```python
from build123d import *

# Parameters (mm, degrees)
SALIENTE_EXTRUIR1_DEPTH = 10
SALIENTE_EXTRUIR2_DEPTH = 5
REDONDEO1_R             = 5
CORTAR_EXTRUIR2_REACH   = 48.394
CROQUIS4_R              = 1.5
CORTAR_EXTRUIR3_DEPTH   = 5


with BuildPart() as part:
    # Croquis1 → Saliente-Extruir1 (new, symmetric)
    with BuildSketch(Plane(origin=(0, 0, 0), x_dir=(0, 0, -1), z_dir=(1, 0, 0))):
        Polygon((20.5, 0), (0, 0), (-3.1, -9.2), (-3.1, -13.1), (-3.019721522, -15), (0.873328538, -14.835511509), (0.8, -13.1), (6, -13.1), (6, -10.1), (2.7, -10.1), (2.7, -7), (6, -7), (6, -4), (14, -4), (14, -7), (17.3, -7), (17.3, -10.1), (14, -10.1), (14, -13.1), (20.5, -13.1), align=None)
    extrude(amount=SALIENTE_EXTRUIR1_DEPTH, both=True)

    # Croquis1<4> → Saliente-Extruir2 (add, symmetric)
    with BuildSketch(Plane(origin=(0, 0, 0), x_dir=(0, 0, -1), z_dir=(1, 0, 0))):
        Polygon((0.873328538, -14.835511509), (-3.019721522, -15), (-1.94652503, -40.4), (1.94652503, -40.235511509), align=None)
    extrude(amount=SALIENTE_EXTRUIR2_DEPTH, both=True)

    # Redondeo1
    redondeo1_edges = [part.edges().sort_by_distance(p)[0] for p in [
        (-5, -40.317755755, 0),
        (5, -40.317755755, 0),
    ]]
    fillet(redondeo1_edges, radius=REDONDEO1_R - 0.0001)  # a hair under: the kernel refuses the full size

    # Croquis3 → Cortar-Extruir2 (cut, up to next)
    with BuildSketch(Plane(origin=(0, 0, 0), x_dir=(1, 0, 0), z_dir=(0, 1, 0)), mode=Mode.PRIVATE) as cortar_extruir2_sk1:
        with BuildLine():
            Line((-6, 11.75), (6, 11.75))
            ThreePointArc((6, 11.75), (7.5, 10.25), (6, 8.75))
            Line((6, 8.75), (-6, 8.75))
            ThreePointArc((-6, 8.75), (-7.5, 10.25), (-6, 11.75))
        make_face()
    cortar_extruir2_tool1 = extrude(cortar_extruir2_sk1.sketch, amount=-CORTAR_EXTRUIR2_REACH, mode=Mode.PRIVATE) & part.part
    add(cortar_extruir2_tool1.solids().sort_by_distance((0, 0, -10.25))[0], mode=Mode.SUBTRACT)

    # Croquis4 → Cortar-Extruir3 (cut, symmetric)
    with BuildSketch(Plane.XY):
        with Locations(Location((0, -35.404457076, 0), (0, 0, 270))):
            Circle(CROQUIS4_R)
    extrude(amount=CORTAR_EXTRUIR3_DEPTH, both=True, mode=Mode.SUBTRACT)


solid = part.part
```
Geometry: final body of the model. Coordinates: model frame, mm. A direction names the side the tool comes from. Give positions to 0.01 mm unless a question says otherwise; leave off trailing zeros. Order: outer loops, then holes, each group sorted by start corner. A loop starts at its lowest first (then second) coordinate and runs counter-clockwise, first axis right, second up. Notation, with made-up numbers: (11, 11.25) -> (38, 11.25) arc R15 cw to (38, 16.25) -> close; hole circle Ø3 at (-13.5, 5.5). An arc over 180 degrees is marked (long way). Write each question's results on one line, items separated by ' | '. Start each with the question number.
1) Set-up query: faces 4 (the flat face through (0, -7, -16)), 5 (the flat face through (0, -2, -8.75)), 6 (the flat face through (0, -13.1, -3)). Return all of +Z, -Z, +X, -X, +Y, -Y with unobstructed straight access to the full face (end or side cutting, diameter ignored); none if empty.
2) Section A-A (z = -5.25). Return loops of the section in (x, y).
3) Section D-D (x = -2). Return loops of the section in (y, z).
4) Line query: line 1 (Z direction, x = -5.75, y = -13); line 2 (Y direction, x = -7.5, z = -3); line 3 (Y direction, x = -7.25, z = -7.75). Output: solid intervals per line, ascending. Write a range as from..to.
5) Section C-C (y = -34.5). Return loops of the section in (x, z), then the cut area to 3 significant figures.
6) Draft query along X for faces 1 (the flat face through (0, -2, -11.75)), 2 (the flat face through (5, -25, 1)), 3 (the flat face through (0, -13.1, -17)). Return one class per face: pulls with the +X half, pulls with the -X half, needs draft (parallel to the pull), parting line crosses it, or undercut.
7) First-contact query: pin 1 (4 mm diameter, centred on x = -4.5, z = -16.5, fed in from -Y); pin 2 (6 mm diameter, centred on x = 2, y = -27.5, fed in from +Z); pin 3 (1.2 mm diameter, centred on x = 1, y = -2, fed in from +Z). Flat tips, straight axial feed; report the tip coordinate or a pass-through.
8) Section B-B (x = -5.5). Return loops of the section in (y, z), then the cut area to 3 significant figures.
Calculated:
1) face 4: +X, -X | face 5: +Y, -Y | face 6: -Z, +X, -X
2) outline: (-10, -13.1) -> (10, -13.1) -> (10, -10.1) -> (-10, -10.1) -> close; (-10, -7) -> (10, -7) -> (10, 0) -> (-10, 0) -> close
3) outline: (-39.98, 1.96) -> (-39.82, -1.93) -> (-13.1, -0.8) -> (-13.1, -6) -> (-10.1, -6) -> (-10.1, -2.7) -> (-7, -2.7) -> (-7, -6) -> (-4, -6) -> (-4, -8.75) -> (0, -8.75) -> (0, 0) -> (-9.2, 3.1) -> (-13.1, 3.1) -> close; (-13.1, -20.5) -> (0, -20.5) -> (0, -11.75) -> (-4, -11.75) -> (-4, -14) -> (-7, -14) -> (-7, -17.3) -> (-10.1, -17.3) -> (-10.1, -14) -> (-13.1, -14) -> close
4) line 1: -20.5..-14, -6..3.1 | line 2: -13.1..-10.1, -7..0 | line 3: -4..0
5) outline: (-5, -1.7) -> (-1.2, -1.7) -> (-1.2, 2.2) -> (-5, 2.2) -> close; (1.2, -1.7) -> (5, -1.7) -> (5, 2.2) -> (1.2, 2.2) -> close | area: 29.7 mm2
6) face 1: undercut | face 2: pulls with the +X half | face 3: needs draft
7) pin 1: y = -13.1 | pin 2: z = 2.62 | pin 3: z = 0.88
8) outline: (-15, 3.02) -> (-14.84, -0.87) -> (-13.1, -0.8) -> (-13.1, -6) -> (-10.1, -6) -> (-10.1, -2.7) -> (-7, -2.7) -> (-7, -6) -> (-4, -6) -> (-4, -8.75) -> (0, -8.75) -> (0, 0) -> (-9.2, 3.1) -> (-13.1, 3.1) -> close; (-13.1, -20.5) -> (0, -20.5) -> (0, -11.75) -> (-4, -11.75) -> (-4, -14) -> (-7, -14) -> (-7, -17.3) -> (-10.1, -17.3) -> (-10.1, -14) -> (-13.1, -14) -> close | area: 197 mm2
